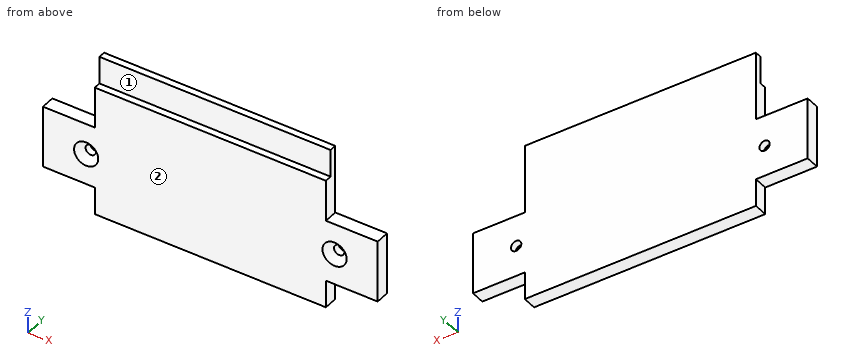
Autodesk Inventor part; units mm, degrees
ref_plane "YZ Plane" through (0, 0, 0) normal (1, 0, 0) x (0, 1, 0)
ref_plane "XZ Plane" through (0, 0, 0) normal (0, 1, 0) x (-1, 0, 0)
ref_plane "XY Plane" through (0, 0, 0) normal (0, 0, 1) x (1, 0, 0)
sketch "Sketch1" plane through (0, 0, 0) normal (0, 1, 0) x (-1, 0, 0)
  line L0 (-33.5, -23) -> (33.5, -23)
  line L1 (33.5, -23) -> (33.5, 23)
  line L2 (33.5, 23) -> (-33.5, 23)
  line L3 (-33.5, 23) -> (-33.5, -23)
  line L4 (-33.5, -23) -> (33.5, 23) construction
  line L5 (33.5, -23) -> (-33.5, 23) construction
  line L6 (33.5, 3) -> (48.5, 3)
  line L7 (48.5, 3) -> (48.5, -15)
  line L8 (48.5, -15) -> (33.5, -15)
  line L9 (33.5, -15) -> (33.5, 3)
  line L10 (-33.5, 3) -> (-48.5, 3)
  line L11 (-48.5, 3) -> (-48.5, -15)
  line L12 (-48.5, -15) -> (-33.5, -15)
  line L13 (-33.5, -15) -> (-33.5, 3)
  point P0 (0, 0)
  point P1 (-33.5, 3)
  dimension "d0" = 67
  dimension "d1" = 46
  dimension "d2" = 97
  dimension "d5" = 8
  dimension "d6" = 18
extrude "Extrusion1" add sketch "Sketch1" along normal blind 4
sketch "Sketch2" plane through (0, 0, 0) normal (0, -1, 0) x (1, 0, 0)
  line L0 (-33.5, 23) -> (33.5, 23)
  line L1 (33.5, 23) -> (33.5, 3)
  line L2 (-33.5, 23) -> (33.5, 23)
  line L3 (33.5, 23) -> (33.5, 15)
  line L4 (33.5, 15) -> (-33.5, 15)
  line L5 (-33.5, 15) -> (-33.5, 23)
  point P0 (0, 0)
  dimension "d7" = 8
extrude "Extrusion2" cut sketch "Sketch2" against normal blind 2
sketch "Sketch3" plane through (0, 0, 0) normal (0, -1, 0) x (1, 0, 0)
  circle A0 centre (-36, -6) radius 1.5
  circle A1 centre (36, -6) radius 1.5
  line L0 (48.5, -15) -> (33.5, -15)
  line L1 (48.5, 3) -> (48.5, -15)
  line L2 (-48.5, -15) -> (-48.5, 3)
  line L3 (-33.5, -15) -> (-48.5, -15)
  point P0 (0, 0)
  dimension "d10" = 9
  dimension "d11" = 12.5
  dimension "d12" = 12.5
  dimension "d13" = 9
  dimension "d14" = 3
extrude "Extrusion3" cut sketch "Sketch3" against normal through all
chamfer "Chamfer1" distance 2 angle 45 2 edges at (34.5, 0, -6) (-37.5, 0, -6)
properties part number "WeightBack" material "Lead"
Input: part model. Units: mm. Frame: model coordinates. Face numbers are marked on the shaded views. A direction names the side the tool comes from. Give positions to 0.01 mm unless a question says otherwise; leave off trailing zeros. Order: outer loops, then holes, each group sorted by start corner. A loop starts at its lowest first (then second) coordinate and runs counter-clockwise, first axis right, second up. Notation, with made-up numbers: (34, -16.75) - (49, -16.75) arc R21 cw to (49, -1.75) - close; hole circle Ø1 at (50, -18.5). An arc over 180 degrees is marked (long way). One line per item, written item: value.
1. Reachability of the marked faces 1 and 2 from +Z, -Z, +X, -X, +Y, -Y: full face, straight path, thin tool, end or side. Return the list, or none.
Determined:
face 1: +Z, +X, -X, -Y
face 2: +Z, -Z, +X, -X, -Y
2. Cut plane D-D, the plane z = 14. Output: boundary loops of the cut face in (x, y), and give its area (3 significant figures).
Determined:
outline: (-33.5, 0) - (33.5, 0) - (33.5, 4) - (-33.5, 4) - close
area: 268 mm2
3. Cut plane A-A, the plane z = -6. Output: boundary loops of the cut face in (x, y), and give its area (3 significant figures).
Determined:
outline: (-48.5, 0) - (-39.5, 0) - (-37.5, 2) - (-37.5, 4) - (-48.5, 4) - close; (-34.5, 2) - (-32.5, 0) - (32.5, 0) - (34.5, 2) - (34.5, 4) - (-34.5, 4) - close; (37.5, 2) - (39.5, 0) - (48.5, 0) - (48.5, 4) - (37.5, 4) - close
area: 356 mm2
4. Pin query (flat end, axial travel): pin 1 Ø1.2 at (y, z) = (1, 15) entering from -X; pin 2 Ø1.6 at (x, y) = (-4, 1) entering from +Z; pin 3 Ø1.2 at (y, z) = (1, -18) entering from +X; pin 4 Ø2.5 at (x, z) = (-36, -6) entering from +Y. Return the tip coordinate at first contact, or that it passes through.
Determined:
pin 1: x = -33.5
pin 2: z = 15
pin 3: x = 33.5
pin 4: through
5. Cut plane B-B, the plane x = 36. Output: boundary loops of the cut face in (y, z), and give its area (3 significant figures).
Determined:
outline: (0, -15) - (4, -15) - (4, -7.5) - (2, -7.5) - (0, -9.5) - close; (0, -2.5) - (2, -4.5) - (4, -4.5) - (4, 3) - (0, 3) - close
area: 56.0 mm2
6. Cut plane C-C, the plane x = -1.5. Output: boundary loops of the cut face in (y, z).
Determined:
outline: (0, -23) - (4, -23) - (4, 23) - (2, 23) - (2, 15) - (0, 15) - close
7. Line query: probe 1 along Z at (x, y) = (36, 2.65); probe 2 along X at (y, z) = (2.55, -18); probe 3 along Z at (x, y) = (-12, 1.8). Output: solid intervals per line, ascending.
Determined:
probe 1: -15 to -7.5, -4.5 to 3
probe 2: -33.5 to 33.5
probe 3: -23 to 15
